```python
from build123d import *

# Parameters (mm, degrees)
F0_W     = 1.5
F0_H     = 17
F1_DEPTH = 20
F2_R     = 4
F4_D     = 3.5
F0_W_2   = 22.978194
F6_D     = 35


with BuildPart() as f1:
    # F0 (on Front) → F1 (new body, symmetric)
    with BuildSketch(Plane.XZ):
        with Locations((-19.25, 0)):
            Rectangle(F0_W, F0_H)
        Polygon((0, 10), (-20, 10), (-20, 8.5), (-18.5, 8.5), (-18.5, -8.5), (-20, -8.5), (-20, -10), (20, -10), (20, 10), align=None)
    extrude(amount=F1_DEPTH, both=True)

    # F2
    f2_edges = [f1.edges().sort_by_distance(p)[0] for p in [
        (-20, -20, 0),
        (20, -20, 0),
        (20, 20, 0),
        (-20, 20, 0),
    ]]
    fillet(f2_edges, radius=F2_R)

    # F4 (through all)
    with Locations(Plane(origin=(0, 0, -10), x_dir=(1, 0, 0), z_dir=(0, 0, -1))):
        with Locations((-16, 16), (16, 16), (16, -16), (-16, -16)):
            Hole(F4_D / 2)

    # F0 (on Front) → F5 (revolve, cut)
    with BuildSketch(Plane.XZ):
        with Locations((-31.489097, 0)):
            Rectangle(F0_W_2, F0_H)
    revolve(axis=Axis((0, 0, 9.40158), (0, 0, 1)), mode=Mode.SUBTRACT)

    # F6 (through all)
    with Locations(Plane(origin=(0, 0, -10), x_dir=(1, 0, 0), z_dir=(0, 0, -1))):
        with Locations((0, 0)):
            Hole(F6_D / 2)


solid = f1.part
```
Source: CAD feature listing. Evaluate the final solid. Frame: model axes, mm. A direction names the side the tool comes from. Round coordinates to 2 decimals unless told otherwise and drop trailing zeros. Loops run counter-clockwise (first coordinate to the right, second up) from the corner with the lowest first, then second, coordinate; pieces in that order, holes last. Notation, with made-up numbers: M 79,58 L 125,58 A16 cw 125,89 Z; hole C -17,7 d7. An arc over 180 degrees is marked long. Put each result on its own line as item: value.
(1) Section D-D, the plane z = 7.25. Return loops of the section in (x, y).
Solutions:
outline: C 0,0 d40; hole C 0,0 d35
(2) Section A-A, the plane x = -3. Return loops of the section in (y, z).
Solutions:
outline: M -20,-10 L -17.24,-10 L -17.24,10 L -20,10 L -20,8.5 L -19.77,8.5 L -19.77,-8.5 L -20,-8.5 Z; M 17.24,-10 L 20,-10 L 20,-8.5 L 19.77,-8.5 L 19.77,8.5 L 20,8.5 L 20,10 L 17.24,10 Z
(3) Pull-direction query (Z, two-part tool) for faces 1 (the face through (15, 14, 8.5)), 2 (the face through (16.228, 14.265, 9.26)); classes: released by +Z, released by -Z, zero draft, split by the parting line, or undercut.
Solutions:
face 1: undercut
face 2: zero draft
(4) Ray query, line 1 (Y direction, x = -16, z = 9.35); line 2 (Z direction, x = -17.5, y = -10); line 3 (Y direction, x = 4, z = -1.5). Return the intervals inside material, ascending. Write a range as [from, to].
Solutions:
line 1: [-20, -17.75], [-14.25, -7.09], [7.09, 14.25], [17.75, 20]
line 2: [-10, -8.5], [8.5, 10]
line 3: [-19.6, -17.04], [17.04, 19.6]
(5) First-contact query: pin 1 (4 mm diameter, centred on x = -6.5, z = -3.5, fed in from -Y); pin 2 (3 mm diameter, centred on x = 16, y = -16, fed in from -Z); pin 3 (2 mm diameter, centred on x = -9.5, z = 3, fed in from +Y); pin 4 (3 mm diameter, centred on y = -4.5, z = -6, fed in from +X). Flat tips, straight axial feed; report the tip coordinate or a pass-through.
Solutions:
pin 1: y = -19.49
pin 2: through
pin 3: y = 18.1
pin 4: x = 19.77
(6) Section B-B, the plane y = 5. Return loops of the section in (x, z).
Solutions:
outline: M -20,-10 L -16.77,-10 L -16.77,10 L -20,10 L -20,8.5 L -19.36,8.5 L -19.36,-8.5 L -20,-8.5 Z; M 16.77,-10 L 20,-10 L 20,-8.5 L 19.36,-8.5 L 19.36,8.5 L 20,8.5 L 20,10 L 16.77,10 Z
(7) Section C-C, the plane y = 16.5. State how many separate pieces and enclosed holes the cut face has, and give its area (3 significant figures).
Solutions:
separate pieces: 6
enclosed holes: 0
area: 251 mm²
(8) Access query for faces 3 (the face through (4.336, 19.524, 0.119)), 4 (the face through (15, -14, -8.5)), 5 (the face through (15, 14, -8.5)), 6 (the face through (-14.4, -14.5, -8.5)). Directions: +Z, -Z, +X, -X, +Y, -Y. A direction counts if a zero-diameter tool reaches every point of the face in a straight line with its end or side. Return the directions, or none.
Solutions:
face 3: none
face 4: +X, -Y
face 5: +X, +Y
face 6: -X, -Y
